Autodesk Inventor part; units mm, degrees
ref_plane "YZ Plane" through (0, 0, 0) normal (1, 0, 0) x (0, 1, 0)
ref_plane "XZ Plane" through (0, 0, 0) normal (0, 1, 0) x (-1, 0, 0)
ref_plane "XY Plane" through (0, 0, 0) normal (0, 0, 1) x (1, 0, 0)
sketch "Block1" plane through (0, 0, 0) normal (0, 0, 1) x (1, 0, 0)
  arc A0 (-75.921, -24.9) -> (77.3822, -19.9) centre (0, 0) ccw
  line L0 (-75.921, -24.9) -> (-109.6494, -24.9)
  line L1 (-109.6494, -24.9) -> (-109.6494, -5.1)
  line L2 (-109.6494, -5.1) -> (-49.8397, -5.1)
  arc A1 (-49.8397, -5.1) -> (-49.8397, 5.1) centre (0, 0) ccw
  line L3 (-49.8397, 5.1) -> (-109.6494, 5.1)
  line L4 (-109.6494, 5.1) -> (-109.6494, 24.9)
  line L5 (-109.6494, 24.9) -> (-75.921, 24.9)
  arc A2 (77.3822, 19.9) -> (-75.921, 24.9) centre (0, 0) ccw
  line L6 (77.3822, 19.9) -> (117.3597, 19.9)
  line L7 (117.3597, 19.9) -> (117.3597, -19.9)
  line L8 (117.3597, -19.9) -> (77.3822, -19.9)
  point P0 (-23.1258, 0)
sketch "Sketch1" plane through (0, 0, 0) normal (0, 1, 0) x (-1, 0, 0)
  arc A0 (49.7494, 5) -> (49.7494, -5) centre (0, 0) ccw
  line L0 (49.7494, 5) -> (109.7494, 5)
  line L1 (109.7494, 5) -> (109.7494, 25)
  line L2 (155.1912, 0) -> (-162.9015, 0)
  line L3 (0, -115.4406) -> (0, 115.4406)
  line L4 (109.7494, 25) -> (75.9934, 25)
  line L5 (49.7494, -5) -> (109.7494, -5)
  line L6 (109.7494, -5) -> (109.7494, -25)
  line L7 (109.7494, -25) -> (75.9934, -25)
  line L8 (-77.4597, 20) -> (-117.4597, 20)
  line L9 (-117.4597, 20) -> (-117.4597, 0)
  line L10 (-77.4597, -20) -> (-117.4597, -20)
  line L11 (-117.4597, -20) -> (-117.4597, 0)
  arc A1 (75.9934, 25) -> (-77.4597, 20) centre (0, 0) ccw
  arc A2 (-77.4597, -20) -> (75.9934, -25) centre (0, 0) ccw
  point P0 (43.3013, 25)
  point P1 (43.3013, -25)
  dimension "d0" = 100
  dimension "d4" = 5
  dimension "d5" = 20
  dimension "d13" = 20
  dimension "d14" = 40
  dimension "d20" = 60
extrude "Extrusion1" add sketch "Sketch1" along normal blind 30 contours A0 L3 A1 L4 L1 L0 | A0 L2 L9 L8 A1 L3 | A0 L3 A2 L10 L11 L2 | A0 L5 L6 L7 A2 L3
sketch "Sketch3" plane through (-109.7494, 0, 25) normal (0, 0, 1) x (1, 0, 0)
  circle A0 centre (15, 15) radius 5
  line L0 (0, 0) -> (33.756, 0)
  line L1 (0, 0) -> (0, 30)
  point P0 (109.7494, 0)
  dimension "d8" = 10
  dimension "d9" = 15
  dimension "d10" = 15
extrude "Extrusion2" cut sketch "Sketch3" against normal through all
sketch "Sketch4" plane through (117.4597, 0, -20) normal (0, 0, -1) x (-1, 0, 0)
  circle A0 centre (15, 15) radius 5
  line L0 (0, 0) -> (0, 30)
  line L1 (0, 30) -> (40, 30)
  point P0 (117.4597, 0)
  dimension "d15" = 10
  dimension "d16" = 15
  dimension "d17" = 15
extrude "Extrusion3" cut sketch "Sketch4" against normal through all
sketch "Sketch5" plane through (0, 0, 0) normal (0, -1, 0) x (1, 0, 0)
  line L0 (117.4597, 20) -> (117.4597, -20)
  line L1 (77.4597, 20) -> (117.4597, 20)
  arc A0 (77.4597, 20) -> (-75.9934, 25) centre (0, 0) ccw
  line L2 (-109.7494, 25) -> (-75.9934, 25)
  line L3 (-109.7494, 5) -> (-109.7494, 25)
  line L4 (-49.7494, 5) -> (-109.7494, 5)
  arc A1 (-49.7494, -5) -> (-49.7494, 5) centre (0, 0) ccw
  line L5 (-109.7494, -5) -> (-49.7494, -5)
  line L6 (-109.7494, -25) -> (-109.7494, -5)
  line L7 (-75.9934, -25) -> (-109.7494, -25)
  arc A2 (-75.9934, -25) -> (77.4597, -20) centre (0, 0) ccw
  line L8 (117.4597, -20) -> (77.4597, -20)
sketch "DXF" plane through (0, 0, 0) normal (0, 1, 0) x (-1, 0, 0)
  point P0 (0, 0)
equation "\"d0\" = Grip"
properties part number "mallet_holder"
Geometry check sheet. Reference: the model listing, model coordinates, mm. A direction names the side the tool comes from. Round coordinates to 2 decimals unless told otherwise and drop trailing zeros. Order: outer loops, then holes, each group sorted by start corner. A loop starts at its lowest first (then second) coordinate and runs counter-clockwise, first axis right, second up. Notation, with made-up numbers: (48, -15) - (78, -15) arc R17 cw to (78, 1) - close; hole circle Ø3 at (37, 83). An arc over 180 degrees is marked (long way). Use a Markdown table: item, result. Add a question column.
1) Thickness scan on line 1 along Z through (x, y) = (0, 11); line 2 along X through (y, z) = (11.75, -16.5); line 3 along Z through (x, y) = (-38, 16.5). Record the ranges inside material, lowest first.
2) Section check D-D (z = 0). Record the cut outline in (x, y), then the cut area to 3 significant figures.
3) Section check B-B (y = 24.75). Record the cut outline in (x, z).
4) Section check C-C (z = -38). Record the cut outline in (x, y), then the cut area to 3 significant figures.
5) Gauge pin test, flat ends, axial feed: P1, Ø6, axis at y = 16, z = -32, coming from the +X side; P2, Ø6, axis at y = 22.5, z = -35, coming from the -X side; P3, Ø5, axis at x = -58, y = 23.5, coming from the +Z side; P4, Ø9, axis at x = 102.46, y = 15, coming from the -Z side. Record the tip position at first contact, or that the pin passes through.
6) Set-up check for faces 4 (the flat face through (-89, 15, -25)), 5 (the flat face through (97, 15, 20)), 6 (the flat face through (-79, 15, -5)), 7 (the flat face through (97, 15, -20)), 8 (the flat face through (-89, 15, 25)): record each of +Z, -Z, +X, -X, +Y, -Y from which the full face is reachable in a straight line by a thin tool's end or side.
7) Section check A-A (x = 0). Record the cut outline in (y, z), then the cut area to 3 significant figures.
8) Mould release check, pull along Y, two halves, no side actions. Record for faces 1 (the cylindrical face through (-90.131, 13.085, -14.86)), 2 (the flat face through (117.46, 15, 0)), 3 (the flat face through (56, 30, 1)): released by +Y, released by -Y, zero draft, split by the parting line, or undercut.
Established:
| question | item | result |
|---|---|---|
| 1 | line 1 | -80 to -50, 50 to 80 |
| 1 | line 2 | -109.75 to -98.55, -90.95 to -47.2, 47.2 to 98.66, 106.26 to 117.46 |
| 1 | line 3 | -70.4 to -32.5, 32.5 to 70.4 |
| 2 | outline | (50, 0) - (117.46, 0) - (117.46, 30) - (50, 30) - close; hole circle Ø10 at (102.46, 15) |
| 2 | area | 1,950 mm2 |
| 3 | outline | (-109.75, -25) - (-75.99, -25) arc R80 ccw to (77.46, -20) - (117.46, -20) - (117.46, 20) - (77.46, 20) arc R80 ccw to (-75.99, 25) - (-109.75, 25) - (-109.75, 5) - (-49.75, 5) arc R50 cw (long way) to (-49.75, -5) - (-109.75, -5) - close |
| 4 | outline | (-70.4, 0) - (-32.5, 0) - (-32.5, 30) - (-70.4, 30) - close; (32.5, 0) - (70.4, 0) - (70.4, 30) - (32.5, 30) - close |
| 4 | area | 2,270 mm2 |
| 5 | P1 | x = 74.56 |
| 5 | P2 | x = -73.32 |
| 5 | P3 | z = 57.62 |
| 5 | P4 | through |
| 6 | face 4 | -Z, -X, +Y, -Y |
| 6 | face 5 | +Z, +X, +Y, -Y |
| 6 | face 6 | -X, +Y, -Y |
| 6 | face 7 | -Z, +X, +Y, -Y |
| 6 | face 8 | +Z, -X, +Y, -Y |
| 7 | outline | (0, -80) - (30, -80) - (30, -50) - (0, -50) - close; (0, 50) - (30, 50) - (30, 80) - (0, 80) - close |
| 7 | area | 1,800 mm2 |
| 8 | face 1 | undercut |
| 8 | face 2 | zero draft |
| 8 | face 3 | released by +Y |
